Design review of the part built by this model. Coordinates are the model's own, in mm. Coordinates: 2 decimals unless noted, no trailing zeros. Order: outer loops, then holes, each group sorted by start corner. A loop starts at its lowest first (then second) coordinate and runs counter-clockwise, first axis right, second up. Notation, with made-up numbers: (58, 37.25) -> (65, 37.25) arc R27 ccw to (65, 74.25) -> close; hole circle Ø11 at (51.5, 29.25). An arc over 180 degrees is marked (long way). Write item = value, one per line.
```python
from build123d import *

# Parameters (mm, degrees)
SKETCH2_R           = 30
BOSS_EXTRUDE1_DEPTH = 10
CHAMFER1_SIZE       = 2
SKETCH3_R           = 16
CUT_EXTRUDE1_DEPTH  = 10


with BuildPart() as part:
    # Sketch2 → Boss-Extrude1 (new body)
    with BuildSketch(Plane(origin=(0, 0, 0), x_dir=(0, 0, -1), z_dir=(1, 0, 0))):
        Circle(SKETCH2_R)
    extrude(amount=BOSS_EXTRUDE1_DEPTH)

    # Chamfer1
    chamfer1_edges = [part.edges().sort_by_distance(p)[0] for p in [
        (10, 0, 30),
    ]]
    chamfer(chamfer1_edges, length=CHAMFER1_SIZE)

    # Sketch3 → Cut-Extrude1 (cut)
    with BuildSketch(Plane(origin=(10, 0, 0), x_dir=(0, 0, -1), z_dir=(1, 0, 0))):
        Circle(SKETCH3_R)
    extrude(amount=-CUT_EXTRUDE1_DEPTH, mode=Mode.SUBTRACT)


solid = part.part
```
(1) Insertion check: pin 1 (3 mm diameter, centred on x = 5.5, y = 12.5, fed in from -Z); pin 2 (2 mm diameter, centred on x = 2.5, y = 3, fed in from -Z); pin 3 (1.5 mm diameter, centred on x = 7, z = 19, fed in from +Y). Each pin has a flat end and moves straight along its axis. Give the tip position at first contact, or say it passes through.
Report:
pin_1 = -27.91
pin_2 = -29.93
pin_3 = 23.81
(2) We need section A-A (z = 0). Write out the cut boundary in (x, y).
Report:
outline = (0, -30) -> (8, -30) -> (10, -28) -> (10, -16) -> (0, -16) -> close; (0, 16) -> (10, 16) -> (10, 28) -> (8, 30) -> (0, 30) -> close
(3) We need section C-C (x = 4). Write out the cut boundary in (y, z).
Report:
outline = circle Ø60 at (0, 0); hole circle Ø32 at (0, 0)
(4) For L1, parallel to Y at x = 4.25, z = 0; L2, parallel to Y at x = 3.5, z = 3; L3, parallel to Z at x = 8.5, y = -6.5, list the stretches that pass through material, from the lowest coordinate up.
Report:
L1 = -30 to -16, 16 to 30
L2 = -29.85 to -15.72, 15.72 to 29.85
L3 = -28.77 to -14.62, 14.62 to 28.77
(5) The part is to be moulded in two halves that separate along Y. For faces 1 (the flat face through (0, -13, -13)), 2 (the cylindrical face through (3.94, 1.32, 29.97)), 3 (the cylindrical face through (5.07, -15.62, 3.47)), say which applies: released by +Y, released by -Y, zero draft, split by the parting line, or undercut.
Report:
face_1 = zero draft
face_2 = split by the parting line
face_3 = undercut
